The model under review builds one solid part; all positions refer to its coordinate system, in mm. A direction names the side the tool comes from. Coordinates: 2 decimals unless noted, no trailing zeros. Loops run counter-clockwise (first coordinate to the right, second up) from the corner with the lowest first, then second, coordinate; pieces in that order, holes last. Notation, with made-up numbers: M 48.25,14.5 L 57.25,14.5 A20 ccw 57.25,23.5 Z; hole C 29,-27 d3. An arc over 180 degrees is marked long. Return JSON: item names as keys, results as strings.
```python
from build123d import *

# Parameters (mm, degrees)
F1_DEPTH = 3.175
F2_W     = 3.175
F2_H     = 304.8
F3_DEPTH = 22.225
F4_W     = 171.45
F4_H     = 3.175
F6_DEPTH = 12.7
F5_W     = 171.45
F5_H     = 3.175
F7_DEPTH = 12.7
F8_W     = 603.25
F8_H     = 3.175
F9_DEPTH = 22.225


with BuildPart() as f1:
    # F0 (on Top) → F1 (new body)
    with BuildSketch(Plane.XY):
        with BuildLine():
            Line((0, 304.8), (0, 0))
            Line((0, 0), (609.6, 0))
            Line((609.6, 0), (609.6, 304.8))
            Line((609.6, 304.8), (508, 304.8))
            Line((508, 304.8), (488.389272, 245.967815))
            ThreePointArc((488.389272, 245.967815), (479.144357, 233.394448), (464.292716, 228.6))
            Line((464.292716, 228.6), (196.107284, 228.6))
            ThreePointArc((196.107284, 228.6), (181.255643, 233.394448), (172.010728, 245.967815))
            Line((172.010728, 245.967815), (152.4, 304.8))
            Line((152.4, 304.8), (0, 304.8))
        make_face()
    extrude(amount=F1_DEPTH)

    # F2 (on face) → F3 (join)
    with BuildSketch(Plane.XY):
        with Locations((1.5875, 152.4)):
            Rectangle(F2_W, F2_H)
        with Locations((608.0125, 152.4)):
            Rectangle(F2_W, F2_H)
    extrude(amount=-F3_DEPTH)

    # F4 (on face) → F6 (join)
    with BuildSketch(Plane(origin=(606.425, 0, 0), x_dir=(0, -1, 0), z_dir=(-1, 0, 0))):
        with Locations((-219.075, -20.6375)):
            Rectangle(F4_W, F4_H)
    extrude(amount=F6_DEPTH)

    # F5 (on face) → F7 (join)
    with BuildSketch(Plane.YZ.offset(3.175)):
        with Locations((219.075, -20.6375)):
            Rectangle(F5_W, F5_H)
    extrude(amount=F7_DEPTH)

    # F8 (on face) → F9 (join, through all)
    with BuildSketch(Plane(origin=(0, 0, 0), x_dir=(1, 0, 0), z_dir=(0, 0, -1))):
        with Locations((304.8, -131.7625)):
            Rectangle(F8_W, F8_H)
    extrude(amount=F9_DEPTH)


solid = f1.part
```
1. The part is to be moulded in two halves that separate along Z. For faces 5 (the face through (303, 0, 2)), 6 (the face through (301, 66, 0)), 7 (the face through (600, 220, -19.05)), say which applies: released by +Z, released by -Z, zero draft, split by the parting line, or undercut.
Check values:
{"face 5": "zero draft", "face 6": "released by -Z", "face 7": "undercut"}
2. To check wall thickness, follow line 1 (X direction, y = 150.5, z = -11) (3 decimals); line 2 (Y direction, x = 479.5, z = -13.75) (3 decimals); line 3 (Z direction, x = 380.5, y = 161) (3 decimals). State the ranges of each line that lie inside material, in increasing order.
Check values:
{"line 1": "0 to 3.175, 606.425 to 609.6", "line 2": "130.175 to 133.35", "line 3": "0 to 3.175"}
3. Add section A-A on x = 561.5. Give the boundary of the cut face in (y, z) (3 decimals), plus the area to 3 significant figures.
Check values:
{"outline": "M 0,0 L 130.175,0 L 130.175,-22.225 L 133.35,-22.225 L 133.35,0 L 304.8,0 L 304.8,3.175 L 0,3.175 Z", "area": "1,040 mm²"}
4. Add section C-C on z = -14.25. Give the boundary of the cut face in (x, y) (3 decimals), plus the area to 3 significant figures.
Check values:
{"outline": "M 0,0 L 3.175,0 L 3.175,130.175 L 606.425,130.175 L 606.425,0 L 609.6,0 L 609.6,304.8 L 606.425,304.8 L 606.425,133.35 L 3.175,133.35 L 3.175,304.8 L 0,304.8 Z", "area": "3,850 mm²"}
5. Add section D-D on y = 185.5. Give the boundary of the cut face in (x, z) (3 decimals).
Check values:
{"outline": "M 0,-22.225 L 15.875,-22.225 L 15.875,-19.05 L 3.175,-19.05 L 3.175,0 L 606.425,0 L 606.425,-19.05 L 593.725,-19.05 L 593.725,-22.225 L 609.6,-22.225 L 609.6,3.175 L 0,3.175 Z"}
6. Machinability: for faces 1 (the face through (606.425, 64, -11)), 2 (the face through (498.332, 275.796, 1.565)), 3 (the face through (606.425, 218, -9)), 4 (the face through (0, 150, -9)), which of the approach directions +Z, -Z, +X, -X, +Y, -Y give a long, thin tool a straight path to every point of the face, cutting with its end or side? Answer none if there is none.
Check values:
{"face 1": "-Z, -Y", "face 2": "+Z, -Z, +Y", "face 3": "+Y", "face 4": "+Z, -Z, -X, +Y, -Y"}
7. Add section B-B on y = 103.5. Give the boundary of the cut face in (x, z) (3 decimals), plus the area to 3 significant figures.
Check values:
{"outline": "M 0,-22.225 L 3.175,-22.225 L 3.175,0 L 606.425,0 L 606.425,-22.225 L 609.6,-22.225 L 609.6,3.175 L 0,3.175 Z", "area": "2,080 mm²"}
8. Insertion check: pin 1 Ø2 at (x, z) = (123.5, -15.5) entering from +Y; pin 2 Ø2.5 at (y, z) = (228.5, -21.5) entering from -X; pin 3 Ø10 at (x, y) = (65.5, 220) entering from -Z; pin 4 Ø2.5 at (x, z) = (334.5, 1.5) entering from +Y. Each pin has a flat end and moves straight along its axis. Give the tip position at first contact, or say it passes through.
Check values:
{"pin 1": "y = 133.35", "pin 2": "x = 0", "pin 3": "z = 0", "pin 4": "y = 228.6"}
